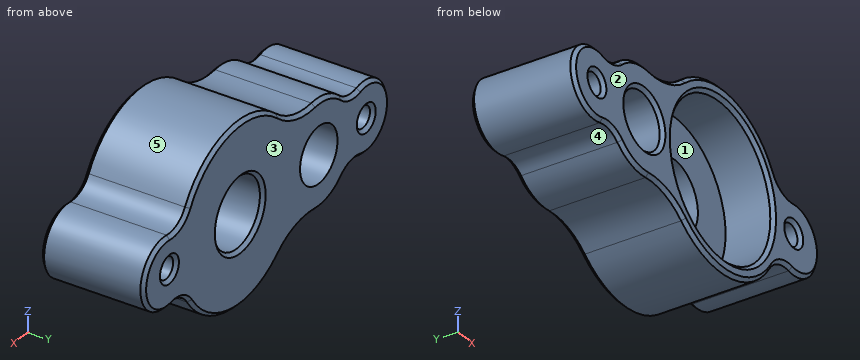
```python
from build123d import *

# Parameters (mm, degrees)
F1_R     = 1.5499996566
F1_R_2   = 4.05
F1_R_3   = 11
F2_DEPTH = 15
F3_R     = 1.5499996566
F3_R_2   = 11
F3_R_3   = 4.05
F3_R_4   = 5
F4_DEPTH = 8
F5_SIZE  = 0.5


# Not quite as in the source:
# - a feature names something its author has since deleted; it is built from what else it names


with BuildPart() as f2:
    # F1 (on offset) → F2 (new body)
    with BuildSketch(Plane.XZ.offset(7.5)):
        with BuildLine():
            ThreePointArc((-16.1097446178, 5.6510393794), (-17.8915523622, 4.7319149036), (-19.8955278727, 4.792831184))
            ThreePointArc((-19.8955278727, 4.792831184), (-26.2950637706, 0.0064660896), (-19.9219776461, -4.815061031))
            ThreePointArc((-19.9219776461, -4.815061031), (-17.917697117, -4.7651791649), (-16.1409768963, -5.694099989))
            ThreePointArc((-16.1409768963, -5.694099989), (-13.3010298936, -7.316379445), (-10.0427278071, -7.6002053168))
            ThreePointArc((-10.0427278071, -7.6002053168), (-5.9542872002, -7.917007121), (-2.3367475524, -9.848099267))
            ThreePointArc((-2.3367475524, -9.848099267), (7.8678117277, -12.7279820224), (16.8033240158, -7.0197971151))
            ThreePointArc((16.8033240158, -7.0197971151), (18.58751675, -5.5306692402), (20.898442998, -5.2847720721))
            ThreePointArc((20.898442998, -5.2847720721), (26.8344703592, -0.5175206843), (21.1826859269, 4.5835026796))
            ThreePointArc((21.1826859269, 4.5835026796), (18.8897447965, 4.9620083109), (17.1942238361, 6.5513648516))
            ThreePointArc((17.1942238361, 6.5513648516), (8.1466571288, 12.85030216), (-2.4748372324, 9.8975183761))
            ThreePointArc((-2.4748372324, 9.8975183761), (-6.0650144321, 7.9160195357), (-10.1486242942, 7.5420670334))
            ThreePointArc((-10.1486242942, 7.5420670334), (-13.3318829255, 7.2355232201), (-16.1097446178, 5.6510393794))
        make_face()
        with Locations((-21.2950828407, -0.0072984656)):
            Circle(F1_R, mode=Mode.SUBTRACT)
        with Locations((-11.0252965242, -0.0355703814)):
            Circle(F1_R_2, mode=Mode.SUBTRACT)
        with Locations((21.2950848365, -0.0073001884)):
            Circle(F1_R, mode=Mode.SUBTRACT)
        with Locations((5.9747034758, 0.0833180019)):
            Circle(F1_R_3, mode=Mode.SUBTRACT)
    extrude(amount=-F2_DEPTH)

    # F3 (on face) → F4 (join)
    with BuildSketch(Plane(origin=(0, 7.5, 0), x_dir=(-1, 0, 0), z_dir=(0, 1, 0))):
        with BuildLine():
            ThreePointArc((10.1486242942, 7.5420670334), (6.0650144321, 7.9160195357), (2.4748372324, 9.8975183761))
            ThreePointArc((2.4748372324, 9.8975183761), (-8.1466571288, 12.85030216), (-17.1942238361, 6.5513648516))
            ThreePointArc((-17.1942238361, 6.5513648516), (-18.8897447965, 4.9620083109), (-21.1826859269, 4.5835026796))
            ThreePointArc((-21.1826859269, 4.5835026796), (-26.8344703592, -0.5175206843), (-20.898442998, -5.2847720721))
            ThreePointArc((-20.898442998, -5.2847720721), (-18.58751675, -5.5306692402), (-16.8033240158, -7.0197971151))
            ThreePointArc((-16.8033240158, -7.0197971151), (-7.8678117277, -12.7279820224), (2.3367475524, -9.848099267))
            ThreePointArc((2.3367475524, -9.848099267), (5.9542872002, -7.917007121), (10.0427278071, -7.6002053168))
            ThreePointArc((10.0427278071, -7.6002053168), (13.3010298936, -7.316379445), (16.1409768963, -5.694099989))
            ThreePointArc((16.1409768963, -5.694099989), (17.917697117, -4.7651791649), (19.9219776461, -4.815061031))
            ThreePointArc((19.9219776461, -4.815061031), (26.2950637706, 0.0064660896), (19.8955278727, 4.792831184))
            ThreePointArc((19.8955278727, 4.792831184), (17.8915523622, 4.7319149036), (16.1097446178, 5.6510393794))
            ThreePointArc((16.1097446178, 5.6510393794), (13.3318829255, 7.2355232201), (10.1486242942, 7.5420670334))
        make_face()
        with Locations((-21.2950848365, -0.0073001884)):
            Circle(F3_R, mode=Mode.SUBTRACT)
        with Locations((-5.9747034758, 0.0833180019)):
            Circle(F3_R_2, mode=Mode.SUBTRACT)
        with Locations((11.0252965242, -0.0355703814)):
            Circle(F3_R_3, mode=Mode.SUBTRACT)
        with Locations((21.2950828407, -0.0072984656)):
            Circle(F3_R, mode=Mode.SUBTRACT)
        with Locations((-5.9747034758, 0.0833180019)):
            Circle(F3_R_2)
        with Locations((-5.9747034758, 0.0833180019)):
            Circle(F3_R_4, mode=Mode.SUBTRACT)
    extrude(amount=-F4_DEPTH)

    # F5
    f5_edges = [f2.edges().sort_by_distance(p)[0] for p in [
        (-6.065014, -7.5, 7.91602),
        (8.146657, -7.5, 12.850302),
        (18.889745, -7.5, 4.962008),
        (26.83447, -7.5, -0.517521),
        (18.587517, -7.5, -5.530669),
        (7.867812, -7.5, -12.727982),
        (-5.954287, -7.5, -7.917007),
        (-13.30103, -7.5, -7.316379),
        (-17.917697, -7.5, -4.765179),
        (-26.295064, -7.5, 0.006466),
        (-17.891552, -7.5, 4.731915),
        (-13.331883, -7.5, 7.235523),
        (-5.025297, -7.5, 0.083318),
        (-22.845082, -7.5, -0.007298),
        (19.745085, -7.5, -0.0073),
        (8.146657, 7.5, 12.850302),
        (-22.845082, 7.5, -0.007298),
        (10.974703, 7.5, 0.083318),
        (19.745085, 7.5, -0.0073),
        (-15.075297, -7.5, -0.03557),
        (-6.065014, 7.5, 7.91602),
        (-13.331883, 7.5, 7.235523),
        (-17.891552, 7.5, 4.731915),
        (-26.295064, 7.5, 0.006466),
        (-17.917697, 7.5, -4.765179),
        (-13.30103, 7.5, -7.316379),
        (-5.954287, 7.5, -7.917007),
        (7.867812, 7.5, -12.727982),
        (18.587517, 7.5, -5.530669),
        (26.83447, 7.5, -0.517521),
        (18.889745, 7.5, 4.962008),
    ]]
    chamfer(f5_edges, length=F5_SIZE)


solid = f2.part
```
Can you work these out from the model? Positions are in its coordinate system, mm. Face numbers are marked on the shaded views. A direction names the side the tool comes from. Give positions to 0.01 mm unless a question says otherwise; leave off trailing zeros. Loops run counter-clockwise (first coordinate to the right, second up) from the corner with the lowest first, then second, coordinate; pieces in that order, holes last. Notation, with made-up numbers: M -11.75,58.25 L -6.75,58.25 A22 ccw -6.75,86.25 Z; hole C -14.5,-12.75 d4. An arc over 180 degrees is marked long. One line per item, written item: value.
(1) Which directions (+Z, -Z, +X, -X, +Y, -Y) give clear straight access to the entire face, cutting with the end or side of a thin tool? Please do the marked faces 1 and 2.
Returned:
face 1: -Y
face 2: +Z, -Z, +X, -X, -Y
(2) Suppose I cut it at A-A on y = -5.5. List the corners of the cut face in (x, z) for me.
Returned:
outline: M -19.92,-4.82 A4 cw -16.14,-5.69 A7.63 ccw -10.04,-7.6 A10 cw -2.34,-9.85 A12.95 ccw 16.8,-7.02 A4 cw 20.9,-5.28 A5 ccw long 21.18,4.58 A4 cw 17.19,6.55 A12.95 ccw -2.47,9.9 A10 cw -10.15,7.54 A7.63 ccw -16.11,5.65 A4 cw -19.9,4.79 A5 ccw long Z; hole C -21.3,-0.01 d3.1; hole C -11.03,-0.04 d8.1; hole C 5.97,0.08 d22; hole C 21.3,-0.01 d3.1
(3) I need wall thicknesses on line 1 (X direction, y = -2.5, z = -0.5); line 2 (X direction, y = 0.5, z = -1); line 3 (X direction, y = 1.5, z = 3.5). Which ranges of each line are inside material? Lowest first, please.
Returned:
line 1: -26.27 to -22.76, -19.83 to -15.05, -7 to -5.01, 16.96 to 19.83, 22.76 to 26.83
line 2: -26.2 to -22.49, -20.1 to -14.96, -7.09 to 1.09, 10.86 to 20.1, 22.49 to 26.8
line 3: -24.86 to -13, -9.05 to 2.32, 9.63 to 25
(4) Suppose I cut it at B-B on z = -3. Count the separate pieces of the cut face and the enclosed holes in it, plus the area to 3 significant figures.
Returned:
separate pieces: 3
enclosed holes: 0
area: 476 mm^2
(5) Suppose I cut it at C-C on y = 4.75. List the corners of the cut face in (x, z) for me.
Returned:
outline: M -19.92,-4.82 A4 cw -16.14,-5.69 A7.63 ccw -10.04,-7.6 A10 cw -2.34,-9.85 A12.95 ccw 16.8,-7.02 A4 cw 20.9,-5.28 A5 ccw long 21.18,4.58 A4 cw 17.19,6.55 A12.95 ccw -2.47,9.9 A10 cw -10.15,7.54 A7.63 ccw -16.11,5.65 A4 cw -19.9,4.79 A5 ccw long Z; hole C -21.3,-0.01 d3.1; hole C -11.03,-0.04 d8.1; hole C 5.97,0.08 d10; hole C 21.3,-0.01 d3.1
(6) We'd pull the mould along X, two halves only. Please class the marked faces 3, 4 and 5: released by +X, released by -X, zero draft, split by the parting line, or undercut.
Returned:
face 3: zero draft
face 4: undercut
face 5: split by the parting line
(7) Will these pins go through, and if not, where does the flat tip stop? pin 1 (5 mm diameter, centred on x = -17, y = -3, fed in from +Z); pin 2 (3 mm diameter, centred on x = 2.5, y = 5.5, fed in from -Z); pin 3 (1.9 mm diameter, centred on x = 21.3, z = -0.01, fed in from +Y); pin 4 (6 mm diameter, centred on y = 1, z = -6.5, fed in from +X).
Returned:
pin 1: z = 6.76
pin 2: z = -12.72
pin 3: through
pin 4: x = 25.74
